from build123d import *

# Parameters (mm, degrees)
SKETCH1_R                = 24.75
SKETCH1_R_2              = 21.75
BOSS_EXTRUDE1_DEPTH      = 750
SKETCH2_R                = 21.75
SKETCH2_R_2              = 12.5
BOSS_EXTRUDE2_DEPTH      = 5
SKETCH3_R                = 21.75
SKETCH3_R_2              = 12.5
BOSS_EXTRUDE3_DEPTH      = 5
SKETCH4_R                = 12.5
BOSS_EXTRUDE4_DEPTH      = 45
BOSS_EXTRUDE4_DEPTH_BACK = 5
SKETCH5_R                = 12.5
BOSS_EXTRUDE5_DEPTH      = 45
BOSS_EXTRUDE5_DEPTH_BACK = 5


with BuildPart() as part:
    # Sketch1 → Boss-Extrude1 (new body)
    with BuildSketch(Plane.XY):
        Circle(SKETCH1_R)
        Circle(SKETCH1_R_2, mode=Mode.SUBTRACT)
    extrude(amount=BOSS_EXTRUDE1_DEPTH)

    # Sketch2 → Boss-Extrude2 (add)
    with BuildSketch(Plane.XY):
        Circle(SKETCH2_R)
        Circle(SKETCH2_R_2, mode=Mode.SUBTRACT)
    extrude(amount=BOSS_EXTRUDE2_DEPTH)

    # Sketch3 → Boss-Extrude3 (add)
    with BuildSketch(Plane.XY.offset(750)):
        Circle(SKETCH3_R)
        Circle(SKETCH3_R_2, mode=Mode.SUBTRACT)
    extrude(amount=-BOSS_EXTRUDE3_DEPTH)

    # Sketch4 → Boss-Extrude4 (add, two sides)
    with BuildSketch(Plane.XY.offset(750)) as boss_extrude4_sk:
        Circle(SKETCH4_R)
    extrude(amount=BOSS_EXTRUDE4_DEPTH)
    extrude(boss_extrude4_sk.sketch, amount=-BOSS_EXTRUDE4_DEPTH_BACK)

    # Sketch5 → Boss-Extrude5 (add, two sides)
    with BuildSketch(Plane(origin=(0, 0, 0), x_dir=(-1, 0, 0), z_dir=(0, 0, -1))) as boss_extrude5_sk:
        Circle(SKETCH5_R)
    extrude(amount=BOSS_EXTRUDE5_DEPTH)
    extrude(boss_extrude5_sk.sketch, amount=-BOSS_EXTRUDE5_DEPTH_BACK)


solid = part.part
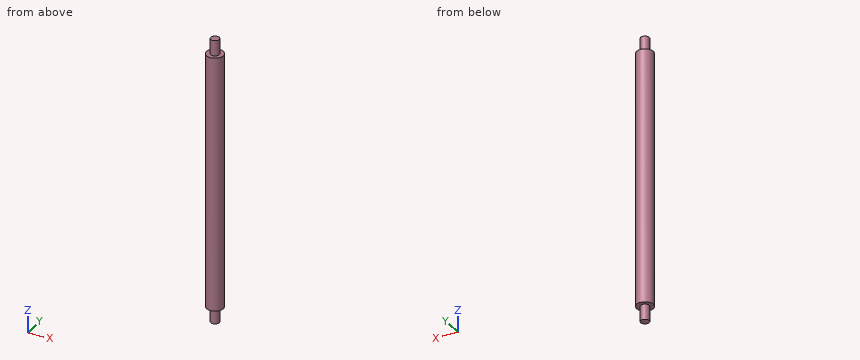
Input: part model. Units: mm. Frame: model coordinates. Give positions to 0.01 mm unless a question says otherwise; leave off trailing zeros. Loops run counter-clockwise (first coordinate to the right, second up) from the corner with the lowest first, then second, coordinate; pieces in that order, holes last. Notation, with made-up numbers: M 2,-36.5 L 28,-36.5 A29 ccw 28,-16.5 Z; hole C 11,25 d5. An arc over 180 degrees is marked long. Use CSV: the item, a comma, the result in double quotes.
(1) Material intervals for L1, parallel to Y at x = 0, z = 300; L2, parallel to Z at x = -16, y = -5.5; L3, parallel to Z at x = -7, y = -1, sorted ascending. Write a range as [from, to].
Outcome:
L1,"y = [-24.75, -21.75], [21.75, 24.75]"
L2,"z = [0, 5], [745, 750]"
L3,"z = [-45, 5], [745, 795]"
(2) Section C-C, the plane z = 636. Return loops of the section in (x, y).
Outcome:
outline,"C 0,0 d49.5; hole C 0,0 d43.5"
(3) Pin query (flat end, axial travel): P1, Ø1.5, axis at x = 1, z = 711, coming from the +Y side; P2, Ø5, axis at y = 6, z = 495, coming from the +X side; P3, Ø12, axis at x = 13.5, y = -14, coming from the -Z side. Return the tip coordinate at first contact, or that it passes through.
Outcome:
P1,"stops at y = 24.75"
P2,"stops at x = 24.5"
P3,"stops at z = 0"
(4) Section A-A, the plane y = 0. Return loops of the section in (x, z).
Outcome:
outline,"M -24.75,0 L -12.5,0 L -12.5,-45 L 12.5,-45 L 12.5,0 L 24.75,0 L 24.75,750 L 12.5,750 L 12.5,795 L -12.5,795 L -12.5,750 L -24.75,750 Z; hole M -21.75,5 L 21.75,5 L 21.75,745 L -21.75,745 Z"
